Can you work these out from the model? Positions are in its coordinate system, mm. Face numbers are marked on the shaded views. Round coordinates to 2 decimals unless told otherwise and drop trailing zeros. Order: outer loops, then holes, each group sorted by start corner. A loop starts at its lowest first (then second) coordinate and runs counter-clockwise, first axis right, second up. Notation, with made-up numbers: (24.25, -13.75) - (53.25, -13.75) arc R22 cw to (53.25, 8.25) - close; hole circle Ø4 at (57.5, -34). An arc over 180 degrees is marked (long way). Write item = value, one per line.
from build123d import *

# Parameters (mm, degrees)
F0_R     = 15.875
F1_DEPTH = 9.525
F2_R     = 29.36875
F3_DEPTH = 22.225
F4_R     = 15.875
F5_DEPTH = 25.4
F6_R     = 9.525
F7_DEPTH = 12.7
F8_R     = 34.925
F9_DEPTH = 9.525
F10_R    = 9.52499


# Not quite as in the source:
# - a fillet or chamfer is up to 0.001 mm smaller than in the source, because OpenCascade refuses the exact size


with BuildPart() as f1:
    # F0 (on Front) → F1 (new body)
    with BuildSketch(Plane.XZ):
        Circle(F0_R)
    extrude(amount=-F1_DEPTH)

    # F2 (on face) → F3 (join)
    with BuildSketch(Plane(origin=(0, 9.525, 0), x_dir=(-1, 0, 0), z_dir=(0, 1, 0))):
        Circle(F2_R)
    extrude(amount=F3_DEPTH)

    # F4 (on face) → F5 (join)
    with BuildSketch(Plane(origin=(0, 31.75, 0), x_dir=(-1, 0, 0), z_dir=(0, 1, 0))):
        Circle(F4_R)
    extrude(amount=F5_DEPTH)

    # F6 (on face) → F7 (join)
    with BuildSketch(Plane(origin=(0, 57.15, 0), x_dir=(-1, 0, 0), z_dir=(0, 1, 0))):
        Circle(F6_R)
    extrude(amount=F7_DEPTH)

    # F8 (on face) → F9 (join)
    with BuildSketch(Plane.XZ):
        Circle(F8_R)
    extrude(amount=F9_DEPTH)

    # F10 (radius 9.525 in the source; OpenCascade refuses exactly that, so slightly less here)
    f10_edges = [f1.edges().sort_by_distance(p)[0] for p in [
        (-34.925, -9.525, 0),
    ]]
    fillet(f10_edges, radius=F10_R)


solid = f1.part
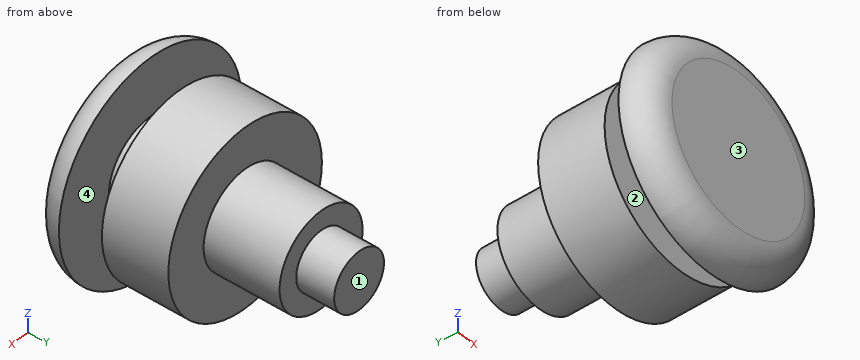
(1) If we section it at C-C (y = 16): Write out the boundary of the cut face in (x, z).
Computed:
outline = circle Ø58.74 at (0, 0)
(2) If I drill on line 1 (Y direction, x = -14, z = -17) (3 decimals); line 2 (X direction, y = 1, z = 0.5); line 3 (Y direction, x = 3.5, z = -14) (3 decimals), over which ranges is the centre line in solid material (lowest first)? Write a range as from..to.
Computed:
line_1 = -9.525..0, 9.525..31.75
line_2 = -15.87..15.87
line_3 = -9.525..57.15
(3) If we section it at D-D (y = 42.5): Write out the boundary of the cut face in (x, z) (3 decimals), plus the area to 3 significant figures.
Computed:
outline = circle Ø31.75 at (0, 0)
area = 792 mm^2
(4) Will these pins go through, and if not, where does the flat tip stop? P1, Ø12, axis at y = 47, z = -5.5, coming from the +X side (3 decimals); P2, Ø3, axis at x = 3, y = 61, coming from the +Z side; P3, Ø5, axis at x = 22, z = -1, coming from the +Y side.
Computed:
P1 = 15.875
P2 = 9.41
P3 = 31.75
(5) Thinking about a two-plate mould opening in Y: for the marked faces 1, 2, 3 and 4, which applies, +Y half, -Y half, draft (parallel to the pull), parting line (faces both ways), or undercut?
Computed:
face_1 = +Y half
face_2 = undercut
face_3 = -Y half
face_4 = undercut
